from build123d import *

# Parameters (mm, degrees)
SKETCH1_R           = 50
BOSS_EXTRUDE1_DEPTH = 35
SKETCH2_R           = 15
BOSS_EXTRUDE2_DEPTH = 220
SKETCH3_W           = 50
SKETCH3_H           = 60
BOSS_EXTRUDE3_DEPTH = 60
CUT_EXTRUDE1_DEPTH  = 81


with BuildPart() as part:
    # Sketch1 → Boss-Extrude1 (new body)
    with BuildSketch(Plane(origin=(0, 0, 0), x_dir=(1, 0, 0), z_dir=(0, 1, 0))):
        Circle(SKETCH1_R)
    extrude(amount=BOSS_EXTRUDE1_DEPTH)

    # Sketch2 → Boss-Extrude2 (add)
    with BuildSketch(Plane(origin=(0, 35, 0), x_dir=(1, 0, 0), z_dir=(0, 1, 0))):
        Circle(SKETCH2_R)
    extrude(amount=BOSS_EXTRUDE2_DEPTH)

    # Sketch3 → Boss-Extrude3 (add)
    with BuildSketch(Plane(origin=(0, 255, 0), x_dir=(1, 0, 0), z_dir=(0, 1, 0))):
        Rectangle(SKETCH3_W, SKETCH3_H)
    extrude(amount=BOSS_EXTRUDE3_DEPTH)

    # Sketch4 → Cut-Extrude1 (cut, through all)
    with BuildSketch(Plane.XY.offset(30)):
        with BuildLine():
            Line((0, 315), (0, 299))
            ThreePointArc((0, 299), (-3.221825407, 291.221825407), (-11, 288))
            Line((-11, 288), (-25, 288))
            Line((-25, 288), (-25, 315))
            Line((-25, 315), (0, 315))
        make_face()
    extrude(amount=-CUT_EXTRUDE1_DEPTH, mode=Mode.SUBTRACT)


solid = part.part
The listing builds one solid part. Answer for the finished solid, in the listing's coordinates (mm). A direction names the side the tool comes from. Give positions to 0.01 mm unless a question says otherwise; leave off trailing zeros. Write each loop counter-clockwise with the first axis right and the second up, starting at its lowest first coordinate (ties: lowest second). Pieces come first, ordered by that corner, then holes.
Item 1: Which of the six approach directions +Z, -Z, +X, -X, +Y, -Y give full straight-line access (tool end or side, diameter ignored) to faces 4 (the flat face through (0, 307, 0)), 5 (the flat face through (5, 278, 30)), 6 (the flat face through (5, 278, -30)), 7 (the flat face through (-12, 35, 10))?
Item 2: Section D-D, the plane y = 278.5 is taken. Write down the section's boundary in (x, z), plus the area to 3 significant figures.
Item 3: Section C-C, the plane x = 3 is taken. Write down the section's boundary in (y, z).
Item 4: Section A-A, the plane z = 19 is taken. Write down the section's boundary in (x, y), plus the area to 3 significant figures.
Item 5: Section B-B, the plane z = 0 is taken. Write down the section's boundary in (x, y), plus the area to 3 significant figures.
Item 6: Flat-ended cylindrical pins translate along their axes: P1, Ø7, axis at x = -20.5, z = -2.5, coming from the +Y side; P2, Ø1, axis at x = 12, y = 126, coming from the -Z side; P3, Ø1.5, axis at x = -14.5, y = 98.5, coming from the +Z side. Find the tip coordinate at first contact, or state that the pin passes through.
Item 7: Determine the mould class of faces 1 (the flat face through (-17, 255, 0)), 2 (the flat face through (-25, 271, 0)), 3 (the flat face through (-18, 288, 0)) for opening direction Y: released by +Y, released by -Y, zero draft, split by the parting line, or undercut.
Item 8: Find the intervals of material crossed by line 1 along Y through (x, z) = (-22, 6); line 2 along Y through (x, z) = (12, -19); line 3 along Y through (x, z) = (1, -31.5), in increasing order.
Completed:
1. face 4: +Z, -Z, -X, +Y
1. face 5: +Z, +X, -X, +Y
1. face 6: -Z, +X, -X, +Y
1. face 7: none
2. outline: (-25, -30) - (25, -30) - (25, 30) - (-25, 30) - close
2. area: 3,000 mm2
3. outline: (0, -49.91) - (35, -49.91) - (35, -14.7) - (255, -14.7) - (255, -30) - (315, -30) - (315, 30) - (255, 30) - (255, 14.7) - (35, 14.7) - (35, 49.91) - (0, 49.91) - close
4. outline: (-46.25, 0) - (46.25, 0) - (46.25, 35) - (-46.25, 35) - close; (-25, 255) - (25, 255) - (25, 315) - (0, 315) - (0, 299) arc R11 cw to (-11, 288) - (-25, 288) - close
4. area: 5,590 mm2
5. outline: (-50, 0) - (50, 0) - (50, 35) - (15, 35) - (15, 255) - (25, 255) - (25, 315) - (0, 315) - (0, 299) arc R11 cw to (-11, 288) - (-25, 288) - (-25, 255) - (-15, 255) - (-15, 35) - (-50, 35) - close
5. area: 12,500 mm2
6. P1: stops at y = 288
6. P2: stops at z = -9.63
6. P3: stops at z = 5.99
7. face 1: undercut
7. face 2: zero draft
7. face 3: released by +Y
8. line 1: y = 0 to 35, 255 to 288
8. line 2: y = 0 to 35, 255 to 315
8. line 3: y = 0 to 35
